Work out the finished part from the listing and answer in its coordinate system (mm). Round coordinates to 2 decimals unless told otherwise and drop trailing zeros. Order: outer loops, then holes, each group sorted by start corner. A loop starts at its lowest first (then second) coordinate and runs counter-clockwise, first axis right, second up. Notation, with made-up numbers: (32.5, 76) -> (78.5, 76) arc R15 cw to (78.5, 105) -> close; hole circle Ø8 at (3.5, 49). An arc over 180 degrees is marked (long way). Use a Markdown table: item, result. Add a question column.
Item 1: A flat-ended cylindrical pin translates along its axis: P1, Ø7, axis at x = 0, z = 320, coming from the +Y side. Find the tip coordinate at first contact, or state that the pin passes through.
Item 2: A cutting plane is placed at A-A, the plane y = 14.5. Determine the outline of the cut face in (x, z).
Item 3: A cutting plane is placed at B-B, the plane z = 176. Determine the outline of the cut face in (x, y).
Item 4: Find the intervals of material crossed by L1, parallel to X at y = -10, z = 245; L2, parallel to X at y = 23, z = 320, in increasing order. Write a range as [from, to].
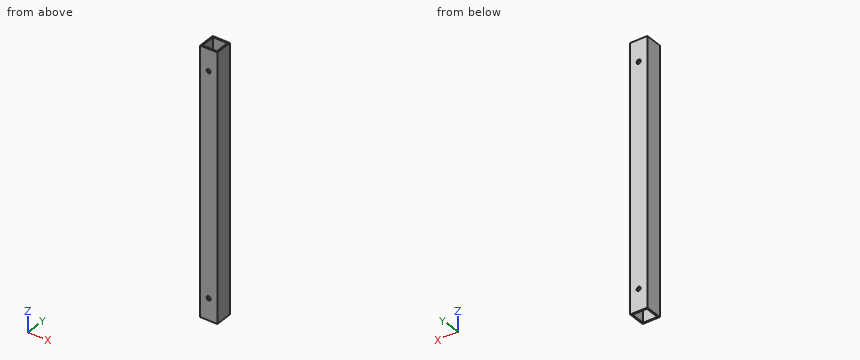
from build123d import *

# Parameters (mm, degrees)
SKETCH_1_W          = 50
SKETCH_1_H          = 50
SKETCH_1_W_2        = 42
SKETCH_1_H_2        = 42
EXTRUDE_1_DEPTH     = 382.5
SKETCH_2_R          = 6
CUT_EXTRUDE_1_DEPTH = 387.563384195


with BuildPart() as part:
    # 草图1 → 凸台-拉伸1 (new, symmetric)
    with BuildSketch(Plane.XY):
        Rectangle(SKETCH_1_W, SKETCH_1_H)
        Rectangle(SKETCH_1_W_2, SKETCH_1_H_2, mode=Mode.SUBTRACT)
    extrude(amount=EXTRUDE_1_DEPTH, both=True)

    # 草图2 → 切除-拉伸1 (cut, through all)
    with BuildSketch(Plane(origin=(0, 25, 0), x_dir=(1, 0, 0), z_dir=(0, 1, 0))):
        with Locations(Location((0, 320, 0), (0, 0, 270))):
            Circle(SKETCH_2_R)
        with Locations(Location((0, -320, 0), (0, 0, 270))):
            Circle(SKETCH_2_R)
    extrude(amount=-CUT_EXTRUDE_1_DEPTH, mode=Mode.SUBTRACT)


solid = part.part
Reported:
| question | item | result |
|---|---|---|
| 1 | P1 | through |
| 2 | outline | (-25, -382.5) -> (-21, -382.5) -> (-21, 382.5) -> (-25, 382.5) -> close; (21, -382.5) -> (25, -382.5) -> (25, 382.5) -> (21, 382.5) -> close |
| 3 | outline | (-25, -25) -> (25, -25) -> (25, 25) -> (-25, 25) -> close; hole (-21, -21) -> (21, -21) -> (21, 21) -> (-21, 21) -> close |
| 4 | L1 | [-25, -21], [21, 25] |
| 4 | L2 | [-25, -6], [6, 25] |
